from build123d import *

# Parameters (mm, degrees)
F0_W     = 20
F0_H     = 30
F1_DEPTH = 3
F2_R     = 1.5
F3_DEPTH = 5


# Not quite as in the source:
# - a feature names something its author has since deleted; it is built from what else it names


with BuildPart() as f1:
    # F0 (on Front) → F1 (new body)
    with BuildSketch(Plane.XZ):
        with Locations((3.3097672276, -12)):
            Rectangle(F0_W, F0_H)
    extrude(amount=F1_DEPTH)

    # F2 (on face) → F3 (join)
    with BuildSketch(Plane.XZ.offset(3)):
        with Locations((-3.6902327724, 0)):
            Circle(F2_R)
    extrude(amount=F3_DEPTH)


solid = f1.part
Can you work these out from the model? Positions are in its coordinate system, mm. A direction names the side the tool comes from. Round coordinates to 2 decimals unless told otherwise and drop trailing zeros. Order: outer loops, then holes, each group sorted by start corner. A loop starts at its lowest first (then second) coordinate and runs counter-clockwise, first axis right, second up. Notation, with made-up numbers: (47, -30) - (74, -30) arc R19 cw to (74, -15) - close; hole circle Ø1 at (80.25, -28.75). An arc over 180 degrees is marked (long way). Answer in a Markdown table with one row per item.
(1) Suppose I cut it at A-A, the plane z = 0. Please give me the cut outline in (x, y).
From the geometry:
| item | result |
|---|---|
| outline | (-6.69, -3) - (-5.19, -3) - (-5.19, -8) - (-2.19, -8) - (-2.19, -3) - (13.31, -3) - (13.31, 0) - (-6.69, 0) - close |
(2) If we mould it in two halves opening along Y, with no side actions, what happens to faces 3 (the face through (-4, -8, 0)), 4 (the face through (3, -1, 3)), 5 (the face through (3, 0, -12))? For each: released by +Y, released by -Y, zero draft, split by the parting line, or undercut.
From the geometry:
| item | result |
|---|---|
| face 3 | released by -Y |
| face 4 | zero draft |
| face 5 | released by +Y |
(3) Which directions (+Z, -Z, +X, -X, +Y, -Y) give clear straight access to the entire face, cutting with the end or side of a thin tool? Please do faces 1 (the face through (3, -1, -27)), 2 (the face through (-2.305, -5.465, -0.575)).
From the geometry:
| item | result |
|---|---|
| face 1 | -Z, +X, -X, +Y, -Y |
| face 2 | -Y |
(4) For P1, Ø2, axis at y = -6.5, z = -1.5, coming from the +X side; P2, Ø4, axis at x = 8, z = -11, coming from the -Y side, each with a flat end and sliding along its axis, tell me the tip position at first contact or that it passes through.
From the geometry:
| item | result |
|---|---|
| P1 | stops at x = -2.28 |
| P2 | stops at y = -3 |
(5) Please list where these lines run through material, in increasing order: L1, parallel to Y at x = -4.25, z = -24.5; L2, parallel to X at y = -3.75, z = 0.25; L3, parallel to X at y = -4.5, z = 0.75. Write a range as from..to.
From the geometry:
| item | result |
|---|---|
| L1 | y = -3..0 |
| L2 | x = -5.17..-2.21 |
| L3 | x = -4.99..-2.39 |
(6) Suppose I cut it at B-B, the plane y = -5.5. Please give me the cut outline in (x, z).
From the geometry:
| item | result |
|---|---|
| outline | circle Ø3 at (-3.69, 0) |
(7) Suppose I cut it at D-D, the plane x = 10. Please give me the cut outline in (y, z).
From the geometry:
| item | result |
|---|---|
| outline | (-3, -27) - (0, -27) - (0, 3) - (-3, 3) - close |
(8) Suppose I cut it at C-C, the plane x = -2.75. Please give me the cut outline in (y, z).
From the geometry:
| item | result |
|---|---|
| outline | (-8, -1.17) - (-3, -1.17) - (-3, -27) - (0, -27) - (0, 3) - (-3, 3) - (-3, 1.17) - (-8, 1.17) - close |
